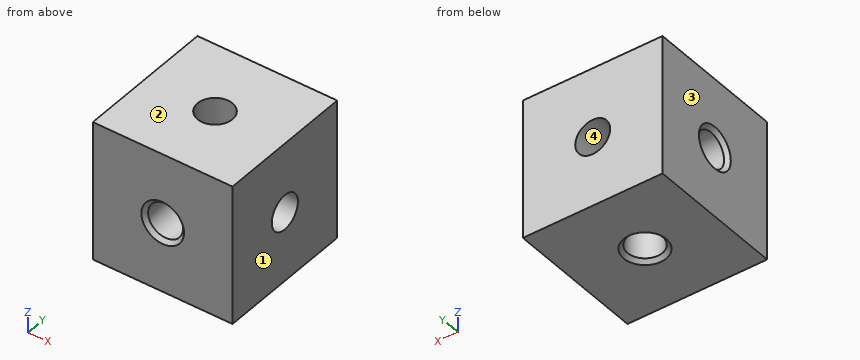
```python
from build123d import *

# Parameters (mm, degrees)
SKETCH_1_W                   = 10
SKETCH_1_H                   = 10
EXTRUDE_1_DEPTH              = 10
HOLE_WIZARD_M3_1_D           = 2.5
HOLE_WIZARD_M3_1_CSINK_D     = 3.05
HOLE_WIZARD_M3_1_CSINK_ANGLE = 90
HOLE_WIZARD_M3_2_D           = 2.5
HOLE_WIZARD_M3_2_CSINK_D     = 3.05
HOLE_WIZARD_M3_2_CSINK_ANGLE = 90
HOLE_WIZARD_M3_3_D           = 2.5
HOLE_WIZARD_M3_3_CSINK_D     = 3.05
HOLE_WIZARD_M3_3_CSINK_ANGLE = 90


with BuildPart() as part:
    # 草图1 → 凸台-拉伸1 (new body)
    with BuildSketch(Plane(origin=(0, 0, 0), x_dir=(1, 0, 0), z_dir=(0, 1, 0))):
        Rectangle(SKETCH_1_W, SKETCH_1_H)
    extrude(amount=EXTRUDE_1_DEPTH)

    # M3 螺纹孔1 (through all)
    with Locations(Plane(origin=(0, 0, 0), x_dir=(-1, 0, 0), z_dir=(0, -1, 0))):
        with Locations((0, 0)):
            CounterSinkHole(HOLE_WIZARD_M3_1_D / 2, HOLE_WIZARD_M3_1_CSINK_D / 2, counter_sink_angle=HOLE_WIZARD_M3_1_CSINK_ANGLE)

    # M3 螺纹孔2 (through all)
    with Locations(Plane(origin=(0, 0, -5), x_dir=(-1, 0, 0), z_dir=(0, 0, -1))):
        with Locations((0, 5)):
            CounterSinkHole(HOLE_WIZARD_M3_2_D / 2, HOLE_WIZARD_M3_2_CSINK_D / 2, counter_sink_angle=HOLE_WIZARD_M3_2_CSINK_ANGLE)

    # M3 螺纹孔3 (through all)
    with Locations(Plane.ZY.offset(5)):
        with Locations((0, 5)):
            CounterSinkHole(HOLE_WIZARD_M3_3_D / 2, HOLE_WIZARD_M3_3_CSINK_D / 2, counter_sink_angle=HOLE_WIZARD_M3_3_CSINK_ANGLE)


solid = part.part
```
Geometry: final body of the model. Coordinates: model frame, mm. Face numbers are marked on the shaded views. Coordinates: 2 decimals unless noted, no trailing zeros. Order: outer loops, then holes, each group sorted by start corner. A loop starts at its lowest first (then second) coordinate and runs counter-clockwise, first axis right, second up.
Item 1: Section query C-C (z = 3.75). Output: boundary loops of the cut face in (x, y).
Answer:
outline: (-5, 0) - (5, 0) - (5, 10) - (-5, 10) - close; hole circle Ø2.5 at (0, 5)
Item 2: Section query D-D (x = 2.5). Output: boundary loops of the cut face in (y, z), then the cut area to 3 significant figures.
Answer:
outline: (0, -5) - (10, -5) - (10, 5) - (0, 5) - close; hole circle Ø2.5 at (5, 0)
area: 95.1 mm2
Item 3: Draft query along X for the marked faces 1, 2, 3 and 4. Return one class per face: released by +X, released by -X, zero draft, split by the parting line, or undercut.
Answer:
face 1: released by +X
face 2: zero draft
face 3: released by -X
face 4: undercut
Item 4: Section query A-A (z = 0). Output: boundary loops of the cut face in (x, y) (3 decimals).
Answer:
outline: (-5, 0) - (-1.525, 0) - (-1.25, 0.275) - (-1.25, 3.75) - (-4.725, 3.75) - (-5, 3.475) - close; (-5, 6.525) - (-4.725, 6.25) - (-1.25, 6.25) - (-1.25, 10) - (-5, 10) - close; (1.25, 0.275) - (1.525, 0) - (5, 0) - (5, 3.75) - (1.25, 3.75) - close; (1.25, 6.25) - (5, 6.25) - (5, 10) - (1.25, 10) - close
Item 5: Section query B-B (y = 5). Output: boundary loops of the cut face in (x, z) (3 decimals).
Answer:
outline: (-5, -5) - (-1.525, -5) - (-1.25, -4.725) - (-1.25, -1.25) - (-4.725, -1.25) - (-5, -1.525) - close; (-5, 1.525) - (-4.725, 1.25) - (-1.25, 1.25) - (-1.25, 5) - (-5, 5) - close; (1.25, -4.725) - (1.525, -5) - (5, -5) - (5, -1.25) - (1.25, -1.25) - close; (1.25, 1.25) - (5, 1.25) - (5, 5) - (1.25, 5) - close
Item 6: Material intervals for line 1 along Z through (x, y) = (3.9, 5); line 2 along Y through (x, z) = (-2.65, 0); line 3 along Y through (x, z) = (-1.75, -0.5), sorted ascending.
Answer:
line 1: z = -5 to -1.25, 1.25 to 5
line 2: y = 0 to 3.75, 6.25 to 10
line 3: y = 0 to 3.85, 6.15 to 10
